The figure shows three views and two pictorial views of one solid part (mm, origin at its lowest corner). Answer the questions. A direction names the side the tool comes from. Coordinates: 2 decimals unless noted, no trailing zeros. Order: outer loops, then holes, each group sorted by start corner. A loop starts at its lowest first (then second) coordinate and runs counter-clockwise, first axis right, second up. Notation, with made-up numbers: (63.25, 44.5) -> (70.25, 44.5) arc R14 ccw to (70.25, 51.5) -> close; hole circle Ø10 at (-14.75, 43.25). An arc over 180 degrees is marked (long way). Write item = value, one per line.
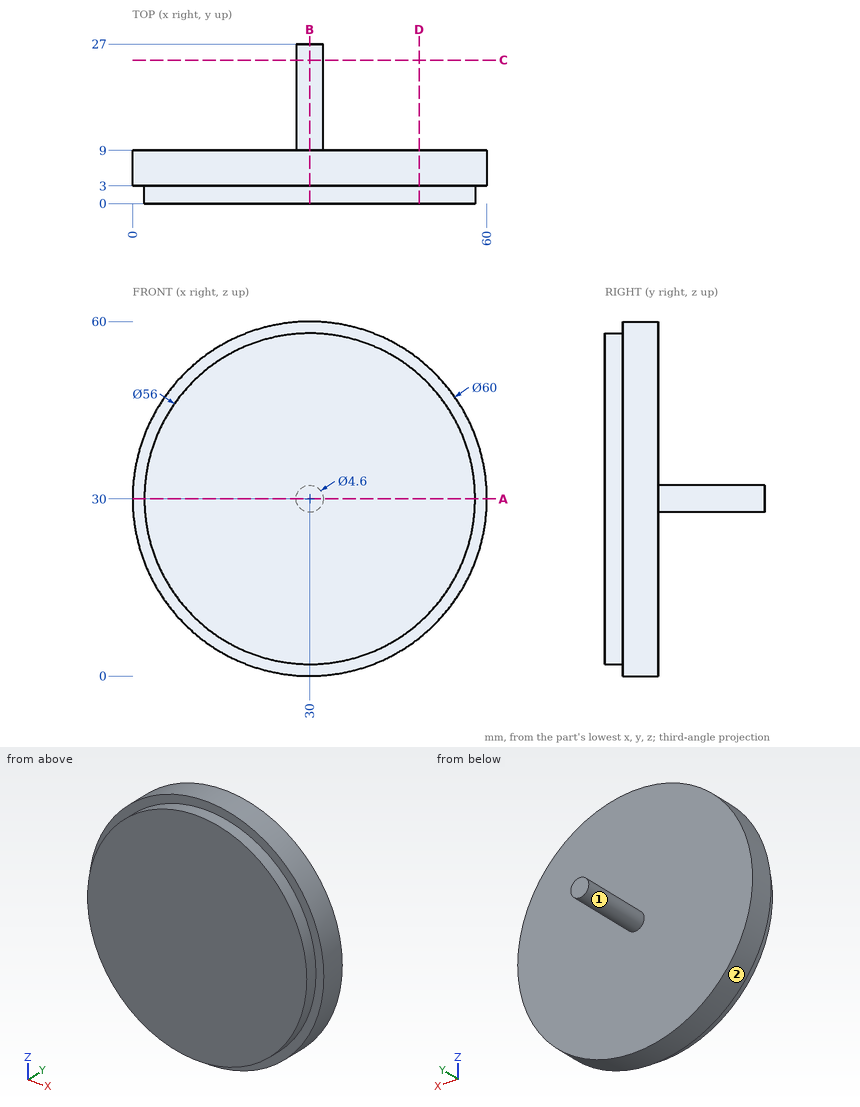
Q1. Find the intervals of material crossed by line 1 along Y through (x, z) = (8.5, 34); line 2 along Y through (x, z) = (46, 5); line 3 along X through (y, z) = (16, 30.5) (3 decimals), in increasing order.
The answers:
line_1 = 0 to 9
line_2 = 3 to 9
line_3 = 27.755 to 32.245
Q2. Section D-D, the plane x = 48.5 is taken. Give the vertices of the cut face in (y, z).
The answers:
outline = (0, 8.98) -> (3, 8.98) -> (3, 6.38) -> (9, 6.38) -> (9, 53.62) -> (3, 53.62) -> (3, 51.02) -> (0, 51.02) -> close
Q3. Section A-A, the plane z = 30 is taken. Give the vertices of the cut face in (x, y), plus the area to 3 significant figures.
The answers:
outline = (0, 3) -> (2, 3) -> (2, 0) -> (58, 0) -> (58, 3) -> (60, 3) -> (60, 9) -> (32.3, 9) -> (32.3, 27) -> (27.7, 27) -> (27.7, 9) -> (0, 9) -> close
area = 611 mm2
Q4. Each of these flat-tipped pins is pushed along its axis until it touches: pin 1 Ø12 at (x, y) = (11, 3) entering from +Z; pin 2 Ø1 at (x, y) = (13, 6.5) entering from -Z; pin 3 Ø3 at (x, y) = (52, 5.5) entering from +Z; pin 4 Ø5 at (x, z) = (27.5, 51) entering from -Y. Where does it stop, or does it pass through?
The answers:
pin_1 = 57.04
pin_2 = 4.95
pin_3 = 51.9
pin_4 = 0
Q5. A tool of negligible diameter and unlimited length cuts with its end or side. For the marked faces 1 and 2, from which of +Z, -Z, +X, -X, +Y, -Y can it reach the whole face along a straight path? Write none if from no direction.
The answers:
face_1 = +Y
face_2 = +Y, -Y
Q6. Section C-C, the plane y = 24.25 is taken. Give the vertices of the cut face in (x, z).
The answers:
outline = circle Ø4.6 at (30, 30)
Q7. Section B-B, the plane x = 30 is taken. Give the vertices of the cut face in (y, z), plus the area to 3 significant figures.
The answers:
outline = (0, 2) -> (3, 2) -> (3, 0) -> (9, 0) -> (9, 27.7) -> (27, 27.7) -> (27, 32.3) -> (9, 32.3) -> (9, 60) -> (3, 60) -> (3, 58) -> (0, 58) -> close
area = 611 mm2
